Source: CAD feature listing. Evaluate the final solid. Frame: model axes, mm. Round coordinates to 2 decimals unless told otherwise and drop trailing zeros. Write each loop counter-clockwise with the first axis right and the second up, starting at its lowest first coordinate (ties: lowest second). Pieces come first, ordered by that corner, then holes. Notation, with made-up numbers: (48, 26.25) -> (92, 26.25) arc R26 cw to (92, 55.25) -> close; hole circle Ø5 at (14, -21.5). An arc over 180 degrees is marked (long way). Put each result on its own line as item: value.
```python
from build123d import *

# Parameters (mm, degrees)
ESBO_O1_W                = 99.1
ESBO_O1_H                = 166.52
RESSALTO_EXTRUS_O1_DEPTH = 5
FILETE1_R                = 3
ESBO_O2_R                = 3.1
CORTE_EXTRUS_O1_DEPTH    = 1.6
ESBO_O3_R                = 3.1
CORTE_EXTRUS_O2_DEPTH    = 1.6
ESBO_O4_R                = 3.1
CORTE_EXTRUS_O3_DEPTH    = 1.6
ESBO_O5_R                = 3.1
CORTE_EXTRUS_O4_DEPTH    = 1.6


with BuildPart() as part:
    # Esboço1 → Ressalto-extrusão1 (new body)
    with BuildSketch(Plane.XY):
        with Locations((5.497464185, 11.397762804)):
            Rectangle(ESBO_O1_W, ESBO_O1_H)
    extrude(amount=RESSALTO_EXTRUS_O1_DEPTH)

    # Filete1
    filete1_edges = [part.edges().sort_by_distance(p)[0] for p in [
        (55.047464185, 11.397762804, 5),
        (5.497464185, 94.657762804, 5),
        (-44.052535815, 11.397762804, 5),
        (5.497464185, -71.862237196, 5),
    ]]
    fillet(filete1_edges, radius=FILETE1_R)

    # Esboço2 → Corte-extrusão1 (cut)
    with BuildSketch(Plane(origin=(0, 0, 0), x_dir=(-1, 0, 0), z_dir=(0, 0, -1))):
        with Locations((-51.497464185, 91.107762804)):
            Circle(ESBO_O2_R)
    extrude(amount=-CORTE_EXTRUS_O1_DEPTH, mode=Mode.SUBTRACT)

    # Esboço3 → Corte-extrusão2 (cut)
    with BuildSketch(Plane(origin=(0, 0, 0), x_dir=(-1, 0, 0), z_dir=(0, 0, -1))):
        with Locations((40.502535815, 91.107762804)):
            Circle(ESBO_O3_R)
    extrude(amount=-CORTE_EXTRUS_O2_DEPTH, mode=Mode.SUBTRACT)

    # Esboço4 → Corte-extrusão3 (cut)
    with BuildSketch(Plane(origin=(0, 0, 0), x_dir=(-1, 0, 0), z_dir=(0, 0, -1))):
        with Locations((-51.497464185, -68.312237196)):
            Circle(ESBO_O4_R)
    extrude(amount=-CORTE_EXTRUS_O3_DEPTH, mode=Mode.SUBTRACT)

    # Esboço5 → Corte-extrusão4 (cut)
    with BuildSketch(Plane(origin=(0, 0, 0), x_dir=(-1, 0, 0), z_dir=(0, 0, -1))):
        with Locations((40.502535815, -68.312237196)):
            Circle(ESBO_O5_R)
    extrude(amount=-CORTE_EXTRUS_O4_DEPTH, mode=Mode.SUBTRACT)


solid = part.part
```
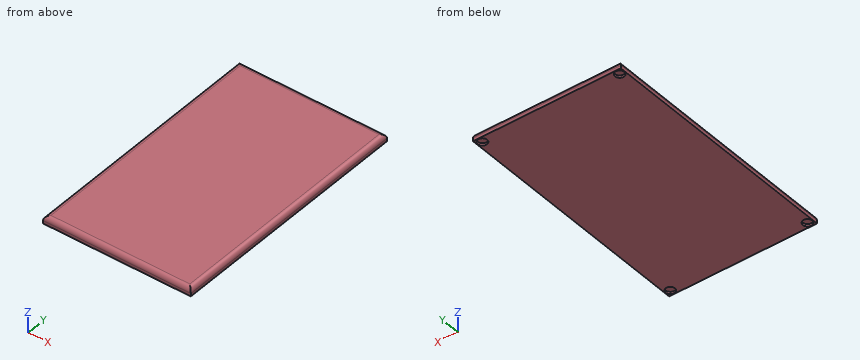
Q1. Cut plane A-A on z = 3.65. Output: boundary loops of the cut face in (x, y), and give its area (3 significant figures).
Ans:
outline: (-43.56, -71.37) -> (54.55, -71.37) -> (54.55, 94.16) -> (-43.56, 94.16) -> close
area: 16,200 mm^2
Q2. Pin query (flat end, axial travel): pin 1 (7 mm diameter, centred on x = 51, y = 92.5, fed in from -Z); pin 2 (1.5 mm diameter, centred on x = -2.5, z = 3, fed in from -Y); pin 3 (2 mm diameter, centred on x = 1.5, z = 3.5, fed in from +Y); pin 4 (5.5 mm diameter, centred on x = -40.5, y = 91.11, fed in from -Z). Return the tip coordinate at first contact, or that it passes through.
Ans:
pin 1: stops at z = 0
pin 2: stops at y = -71.85
pin 3: stops at y = 94.62
pin 4: stops at z = 1.6
Q3. Material intervals for line 1 (Y direction, x = 21, z = 2.1); line 2 (Y direction, x = -9, z = 3.55); line 3 (X direction, y = 37.5, z = 2.45), sorted ascending. Write a range as [from, to].
Ans:
line 1: y = [-71.86, 94.66]
line 2: y = [-71.43, 94.23]
line 3: x = [-44.02, 55.01]
